Here's how the part is built. I have some questions about the finished solid (model axes, mm). A direction names the side the tool comes from. Round coordinates to 2 decimals unless told otherwise and drop trailing zeros. Write each loop counter-clockwise with the first axis right and the second up, starting at its lowest first coordinate (ties: lowest second). Pieces come first, ordered by that corner, then holes. Notation, with made-up numbers: (-20.5, 34.5) -> (6.5, 34.5) arc R27 ccw to (6.5, 64.5) -> close; hole circle Ø10 at (-35.5, 3.5). An arc over 180 degrees is marked (long way). Answer as CSV lines item,"result".
from build123d import *

# Parameters (mm, degrees)
F1_ANGLE    = 315
F2_T2_ANGLE = 359.64
F4_DEPTH    = 2.54


# Not quite as in the source:
# - a fillet or chamfer that OpenCascade refuses, or shapes differently, is made with other operations: its cross-section is extruded or revolved along the edge and cut away or added


with BuildPart() as f1:
    # F0 (on Right) → F1 (revolve)
    with BuildSketch(Plane.YZ):
        Polygon((15.24, 21.59), (0, 21.59), (0, 19.05), (9.7782645518, 19.05), (9.7782645518, 0), (12.7, 0), (12.7, 19.05), (15.24, 19.05), align=None)
    revolve(axis=Axis((0, 0, 20.32), (0, 0, 1)), revolution_arc=F1_ANGLE)

    # F2: fillet of radius 5.08 on 1 edges, made by hand

    # F2_s1 → F2_t2 (revolve, cut)
    with BuildSketch(Plane(origin=(0, 0, 0), x_dir=(0, 0, 1), z_dir=(0.9250772068, -0.3797790955, 0))):
        with BuildLine():
            ThreePointArc((21.59, -10.8405909488), (20.9094090512, -13.3805909488), (19.05, -15.24))
            Line((19.05, -15.24), (21.59, -15.24))
            Line((21.59, -15.24), (21.59, -10.8405909488))
        make_face()
    revolve(axis=Axis((0, 0, 21.59), (0, 0, 1)), revolution_arc=F2_T2_ANGLE, mode=Mode.SUBTRACT)

    # F3 (on face) → F4 (join)
    with BuildSketch(Plane(origin=(0, 0, 19.05), x_dir=(1, 0, 0), z_dir=(0, 0, -1))):
        with BuildLine():
            ThreePointArc((0, -9.7782645518), (2.5003109935, -6.0362847106), (6.9142771728, -6.9142771728))
            Line((6.9142771728, -6.9142771728), (0, 0))
            Line((0, 0), (0, -9.7782645518))
        make_face()
    extrude(amount=-F4_DEPTH)


solid = f1.part
Item 1: Suppose I cut it at A-A, the plane y = 0. List the corners of the cut face in (x, z) for me, then the cut area to 3 significant figures.
Results found:
outline,"(-15.24, 19.05) -> (-12.7, 19.05) -> (-12.7, 0) -> (-9.78, 0) -> (-9.78, 19.05) -> (9.78, 19.05) -> (9.78, 0) -> (12.7, 0) -> (12.7, 19.05) -> (15.24, 19.05) arc R5.08 ccw to (10.84, 21.59) -> (-10.84, 21.59) arc R5.08 ccw to start"
area,"182 mm²"
Item 2: If we mould it in two halves opening along Y, with no side actions, what happens to faces 4 (the flat face through (0, 0, 21.59)), 5 (the cylindrical face through (-5.308, -11.538, 9.658)), 6 (the cylindrical face through (-4.09, -8.88, 9.39))? For each: pulls with the +Y half, pulls with the -Y half, needs draft (parallel to the pull), parting line crosses it, or undercut.
Results found:
face 4,"needs draft"
face 5,"parting line crosses it"
face 6,"undercut"
Item 3: Suppose I cut it at B-B, the plane z = 7.5. List the corners of the cut face in (x, y) for me.
Results found:
outline,"(0, 9.78) -> (0, 12.7) arc R12.7 ccw (long way) to (8.98, 8.98) -> (6.91, 6.91) arc R9.78 cw (long way) to start"
Item 4: For faces 1 (the flat face through (-8, -10.1, 19.05)), 2 (the flat face through (-6.6, -7.5, 0)), 3 (the flat face through (8, 8, 11)), which set-ups out of +Z, -Z, +X, -X, +Y, -Y let a thin tool reach every point of the face, with its end or its side?
Results found:
face 1,"-Z"
face 2,"-Z, +X, -X, +Y, -Y"
face 3,"+Z, -Z, +Y"
Item 5: I need wall thicknesses on L1, parallel to X at y = 0, z = 11.75; L2, parallel to Z at x = -4, y = -8; L3, parallel to Y at x = 8, z = 15.25. Which ranges of each line are inside material? Lowest first, please.
Results found:
L1,"x = -12.7 to -9.78, 9.78 to 12.7"
L2,"z = 19.05 to 21.59"
L3,"y = -9.86 to -5.62, 5.62 to 8"
Item 6: Will these pins go through, and if not, where does the flat tip stop? pin 1 (12 mm diameter, centred on x = 5, z = 15.5, fed in from -Y); pin 2 (4.5 mm diameter, centred on y = 12.5, z = 12.5, fed in from +X); pin 3 (4 mm diameter, centred on x = 8.5, z = 9.5, fed in from -Y).
Results found:
pin 1,"stops at y = -15.24"
pin 2,"stops at x = 0"
pin 3,"stops at y = -10.91"
